Geometry: final body of the model. Coordinates: model frame, mm. A direction names the side the tool comes from. Coordinates: 2 decimals unless noted, no trailing zeros. Order: outer loops, then holes, each group sorted by start corner. A loop starts at its lowest first (then second) coordinate and runs counter-clockwise, first axis right, second up. Notation, with made-up numbers: M 29.5,86.25 L 57.5,86.25 A13 cw 57.5,105.25 Z; hole C 53,-28 d10. An arc over 180 degrees is marked long. Use CSV: the item, a comma, the result in double quotes. Start each with the question number.
1. Section query C-C on z = 4.25. Return the cut outline in (x, y).
2. First-contact query: P1, Ø8.5, axis at y = 23, z = 14, coming from the -X side; P2, Ø4, axis at x = 33.25, y = 33.25, coming from the +Z side; P3, Ø10, axis at x = 9, z = 13, coming from the +Y side; P4, Ø3, axis at x = 31, z = 15, coming from the -Y side. Flat tips, straight axial feed; report the tip coordinate or a pass-through.
3. Section query A-A on y = 2.75. Return the cut outline in (x, z).
4. Material intervals for line 1 (Y direction, x = 2.75, z = 1.9); line 2 (Z direction, x = 2, y = 29.5), sorted ascending.
5. Section query D-D on x = 27.5. Return the cut outline in (y, z).
6. Set-up query: faces 4 (the flat face through (26, 18, 13)), 5 (the cylindrical face through (32.06, 34.16, 2.46)). Return all of +Z, -Z, +X, -X, +Y, -Y with unobstructed straight access to the full face (end or side cutting, diameter ignored); none if empty.
7. Pull-direction query (Y, two-part tool) for faces 1 (the cylindrical face through (31.75, 2.68, 2.46)), 2 (the flat face through (31, 31, 13)), 3 (the flat face through (31, 5, 13)); classes: pulls with the +Y half, pulls with the -Y half, needs draft (parallel to the pull), parting line crosses it, or undercut.
from build123d import *

# Parameters (mm, degrees)
SKETCH_W     = 36
SKETCH_H     = 36
PAD_DEPTH    = 5
SKETCH001_W  = 10
SKETCH001_H  = 26
PAD001_DEPTH = 17
SKETCH002_R  = 1.5
POCKET_DEPTH = 5


with BuildPart() as part:
    # Sketch → Pad (new body)
    with BuildSketch(Plane.XY):
        with Locations((18, 18)):
            Rectangle(SKETCH_W, SKETCH_H)
    extrude(amount=PAD_DEPTH)

    # Sketch001 → Pad001 (new body)
    with BuildSketch(Plane.XY.offset(5)):
        with Locations((31, 18)):
            Rectangle(SKETCH001_W, SKETCH001_H)
    extrude(amount=PAD001_DEPTH)

    # Sketch002 → Pocket (cut)
    with BuildSketch(Plane(origin=(0, 0, 0), x_dir=(1, 0, 0), z_dir=(0, 0, -1))):
        with Locations((2.75, -2.75)):
            Circle(SKETCH002_R)
        with Locations((33.25, -2.75)):
            Circle(SKETCH002_R)
        with Locations((33.25, -33.25)):
            Circle(SKETCH002_R)
        with Locations((2.75, -33.25)):
            Circle(SKETCH002_R)
    extrude(amount=-POCKET_DEPTH, mode=Mode.SUBTRACT)


solid = part.part
Results list:
1,outline,"M 0,0 L 36,0 L 36,36 L 0,36 Z; hole C 2.75,2.75 d3; hole C 2.75,33.25 d3; hole C 33.25,2.75 d3; hole C 33.25,33.25 d3"
2,P1,"stops at x = 26"
2,P2,"stops at z = 5"
2,P3,"passes through"
2,P4,"stops at y = 5"
3,outline,"M 0,0 L 1.25,0 L 1.25,5 L 0,5 Z; M 4.25,0 L 31.75,0 L 31.75,5 L 4.25,5 Z; M 34.75,0 L 36,0 L 36,5 L 34.75,5 Z"
4,line 1,"y = 0 to 1.25, 4.25 to 31.75, 34.75 to 36"
4,line 2,"z = 0 to 5"
5,outline,"M 0,0 L 36,0 L 36,5 L 31,5 L 31,22 L 5,22 L 5,5 L 0,5 Z"
6,face 4,"+Z, -X, +Y, -Y"
6,face 5,"+Z, -Z"
7,face 1,"undercut"
7,face 2,"pulls with the +Y half"
7,face 3,"pulls with the -Y half"
